The model under review builds one solid part; all positions refer to its coordinate system, in mm. A direction names the side the tool comes from. Round coordinates to 2 decimals unless told otherwise and drop trailing zeros. Order: outer loops, then holes, each group sorted by start corner. A loop starts at its lowest first (then second) coordinate and runs counter-clockwise, first axis right, second up. Notation, with made-up numbers: M 61.25,-24.75 L 110.25,-24.75 A23 ccw 110.25,3.25 Z; hole C -15,34.25 d7. An arc over 180 degrees is marked long. Use a Markdown table: item, result. Add a question column.
1. For faces 4 (the flat face through (239, -5.08, 0)), 5 (the cylindrical face through (111.009, 2.48, -7.874)), 6 (the flat face through (-11, 6, -5.08)), 7 (the flat face through (-11, 6, 5.08)), 8 (the flat face through (-12, -5.08, 0)), list the 3-axis set-ups (+Z, -Z, +X, -X, +Y, -Y) from which the entire face can be reached by the end or side of a thin tool; tool diameter is ignored.
2. Insertion check: P1, Ø1, axis at x = 173, z = 5.5, coming from the +Y side; P2, Ø1.5, axis at x = 26.5, z = 3.5, coming from the +Y side; P3, Ø1.4, axis at y = 7.5, z = -3.5, coming from the +X side; P4, Ø3, axis at x = -15.875, z = 0, coming from the +Y side. Each pin has a flat end and moves straight along its axis. Give the tip position at first contact, or say it passes through.
3. Consider section A-A on x = 112.5. State the section outline as (y, z) points (3 decimals), then the cut area to 3 significant figures.
4. The part is to be moulded in two halves that separate along X. For faces 1 (the cylindrical face through (241.12, -0.07, -0.69)), 2 (the cylindrical face through (252.474, -0.071, -0.182)), 3 (the flat face through (-13, 5.08, 0)), say which applies: +X half, -X half, draft (parallel to the pull), parting line (faces both ways), or undercut.
5. To check wall thickness, follow probe 1 along X at (y, z) = (7.4, 0); probe 2 along Z at (x, y) = (5.5, 0.75); probe 3 along X at (y, z) = (-1.5, 0) (3 decimals). State the ranges of each line that lie inside material, in increasing order.
from build123d import *

# Parameters (mm, degrees)
SKETCH1_R                = 8.255
BOSS_EXTRUDE1_DEPTH      = 225.171
BOSS_EXTRUDE2_DEPTH      = 5.08
BOSS_EXTRUDE2_DEPTH_BACK = 5.08
SKETCH2_R                = 3.175
BOSS_EXTRUDE3_DEPTH      = 5.08
BOSS_EXTRUDE3_DEPTH_BACK = 5.08
CUT_EXTRUDE1_DEPTH       = 253.962641167
CUT_EXTRUDE1_DEPTH_BACK  = 253.962641167
SKETCH4_R                = 2.398254968


with BuildPart() as part:
    # Sketch1 → Boss-Extrude1 (new body)
    with BuildSketch(Plane(origin=(0, 0, 0), x_dir=(0, 0, -1), z_dir=(1, 0, 0))):
        Circle(SKETCH1_R)
    extrude(amount=BOSS_EXTRUDE1_DEPTH)

    # Sketch2 → Boss-Extrude2 (add, two sides: drawn at the far end of the back side and taken through both)
    with BuildSketch(Plane(origin=(0, 0, 0), x_dir=(1, 0, 0), z_dir=(0, 1, 0)).offset(-BOSS_EXTRUDE2_DEPTH_BACK)):
        with BuildLine():
            Line((225.171, -8.255), (225.171, 8.255))
            Line((225.171, 8.255), (244.221, 8.255))
            ThreePointArc((244.221, 8.255), (252.476, 0), (244.221, -8.255))
            Line((244.221, -8.255), (225.171, -8.255))
        make_face()
        with Locations(Location((244.221, 0, 0), (0, 0, 270))):
            Circle(SKETCH2_R, mode=Mode.SUBTRACT)
    extrude(amount=BOSS_EXTRUDE2_DEPTH + BOSS_EXTRUDE2_DEPTH_BACK)

    # Sketch3 → Boss-Extrude3 (add, two sides: drawn at the far end of the back side and taken through both)
    with BuildSketch(Plane.XY.offset(-BOSS_EXTRUDE3_DEPTH_BACK)):
        Polygon((0, -8.255), (0, 8.255), (-21.59, 8.255), (-21.59, 5.08), (-3.175, 5.08), (-3.175, -5.08), (-21.59, -5.08), (-21.59, -8.255), align=None)
    extrude(amount=BOSS_EXTRUDE3_DEPTH + BOSS_EXTRUDE3_DEPTH_BACK)

    # Sketch4 → Cut-Extrude1 (cut, two sides: drawn at the far end of the back side and taken through both)
    with BuildSketch(Plane(origin=(0, -5.08, 0), x_dir=(1, 0, 0), z_dir=(0, 1, 0)).offset(-CUT_EXTRUDE1_DEPTH_BACK)):
        with Locations(Location((-15.875, 0, 0), (0, 0, 180))):
            Circle(SKETCH4_R)
    extrude(amount=CUT_EXTRUDE1_DEPTH + CUT_EXTRUDE1_DEPTH_BACK, mode=Mode.SUBTRACT)


solid = part.part
Answer block:
| question | item | result |
|---|---|---|
| 1 | face 4 | +Z, -Z, +X, -Y |
| 1 | face 5 | none |
| 1 | face 6 | -Z, -X, +Y, -Y |
| 1 | face 7 | +Z, -X, +Y, -Y |
| 1 | face 8 | +Z, -Z, -X |
| 2 | P1 | y = 6.57 |
| 2 | P2 | y = 7.78 |
| 2 | P3 | x = 225.17 |
| 2 | P4 | through |
| 3 | outline | C 0,0 d16.51 |
| 3 | area | 214 mm^2 |
| 4 | face 1 | undercut |
| 4 | face 2 | +X half |
| 4 | face 3 | draft |
| 5 | probe 1 | -21.59 to -18.27, -13.48 to 225.17 |
| 5 | probe 2 | -8.22 to 8.22 |
| 5 | probe 3 | -3.175 to 241.046, 247.396 to 252.476 |
